For this review, take the finished solid that the model builds, in its own axes (mm). Give positions to 0.01 mm unless a question says otherwise; leave off trailing zeros. Order: outer loops, then holes, each group sorted by start corner. A loop starts at its lowest first (then second) coordinate and runs counter-clockwise, first axis right, second up. Notation, with made-up numbers: M -26,0 L -5,0 A36 ccw -5,35 Z; hole C 19,87.5 d5. An arc over 180 degrees is marked long. Use CSV: the item, a comma, the result in double quotes. Start each with the question number.
(1) Consider section A-A (z = -1). Write out the cut boundary in (x, y) (3 decimals), and give its area (3 significant figures).
(2) Consider section B-B (x = -23). Write out the cut boundary in (y, z).
(3) Wall thickness on L1, parallel to Y at x = -17.5, z = -0.25 (3 decimals); L2, parallel to Y at x = 17.5, z = -0.4 (3 decimals); L3, parallel to X at y = 5.75, z = -1.2: over which ranges is each line inside the solid? List them lowest first. Write a range as from..to.
```python
from build123d import *

# Parameters (mm, degrees)
BOSS_EXTRUDE1_DEPTH = 1.59
SKETCH4_R           = 1
CUT_EXTRUDE1_DEPTH  = 10
SKETCH5_R           = 1
CUT_EXTRUDE2_DEPTH  = 32.778902593


with BuildPart() as part:
    # Sketch3 → Boss-Extrude1 (new, symmetric)
    with BuildSketch(Plane.XY):
        with BuildLine():
            Line((-17.5, 11.825), (17.5, 11.825))
            ThreePointArc((17.5, 11.825), (29.325, 0), (17.5, -11.825))
            Line((17.5, -11.825), (-17.5, -11.825))
            ThreePointArc((-17.5, -11.825), (-29.325, 0), (-17.5, 11.825))
        make_face()
    extrude(amount=BOSS_EXTRUDE1_DEPTH, both=True)

    # Sketch4 → Cut-Extrude1 (cut)
    with BuildSketch(Plane.XY.offset(1.59)):
        with Locations((-17.5, 5.535)):
            Circle(SKETCH4_R)
        with Locations((-17.5, -5.535)):
            Circle(SKETCH4_R)
    extrude(amount=-CUT_EXTRUDE1_DEPTH, mode=Mode.SUBTRACT)

    # Sketch5 → Cut-Extrude2 (cut, through all)
    with BuildSketch(Plane.XY.offset(1.59)):
        with Locations((17.5, 4.5)):
            Circle(SKETCH5_R)
        with Locations((17.5, -4.5)):
            Circle(SKETCH5_R)
        with BuildLine():
            Line((20, 11.557708467), (20, -11.557708467))
            ThreePointArc((20, -11.557708467), (29.325, 0), (20, 11.557708467))
        make_face()
    extrude(amount=-CUT_EXTRUDE2_DEPTH, mode=Mode.SUBTRACT)


solid = part.part
```
Check result:
1,outline,"M -17.5,-11.825 L 17.5,-11.825 A11.825 ccw 20,-11.558 L 20,11.558 A11.825 ccw 17.5,11.825 L -17.5,11.825 A11.825 ccw Z; hole C -17.5,-5.535 d2; hole C -17.5,5.535 d2; hole C 17.5,-4.5 d2; hole C 17.5,4.5 d2"
1,area,"1,090 mm^2"
2,outline,"M -10.47,-1.59 L 10.47,-1.59 L 10.47,1.59 L -10.47,1.59 Z"
3,L1,"y = -11.825..-6.535, -4.535..4.535, 6.535..11.825"
3,L2,"y = -11.825..-5.5, -3.5..3.5, 5.5..11.825"
3,L3,"x = -27.83..-18.48, -16.52..20"
